Here's how the part is built. I have some questions about the finished solid (model axes, mm). Face numbers are marked on the shaded views. A direction names the side the tool comes from. Round coordinates to 2 decimals unless told otherwise and drop trailing zeros. Order: outer loops, then holes, each group sorted by start corner. A loop starts at its lowest first (then second) coordinate and runs counter-clockwise, first axis right, second up. Notation, with made-up numbers: M 48,63.25 L 59,63.25 A9 cw 59,74.25 Z; hole C -27,-20 d3. An arc over 180 degrees is marked long. Use one line per item in the form item = value. Start each with the question number.
```python
from build123d import *

# Parameters (mm, degrees)
SKETCH1_R                = 34.925
BOSS_EXTRUDE2_DEPTH      = 12.7
CUT_EXTRUDE3_START       = -25.4
CUT_EXTRUDE3_DEPTH       = 25.4
FILLET1_R                = 1.27
FILLET2_R                = 1.27
CIRPATTERN2_COUNT        = 20
FILLET1_OF_CIRPATTERN2_R = 1.27
FILLET2_OF_CIRPATTERN2_R = 1.27
CUT_EXTRUDE4_DEPTH       = 51.660303503
CUT_EXTRUDE4_DEPTH_BACK  = 51.660303503
SKETCH1_4_R              = 2.54
BOSS_EXTRUDE3_DEPTH      = 5.08


# Read off the part's stored shape, not the designer's step: Cut-Extrude3
with BuildPart() as part:
    # Sketch1 → Boss-Extrude2 (new, symmetric)
    with BuildSketch(Plane.XY):
        Circle(SKETCH1_R)
    extrude(amount=BOSS_EXTRUDE2_DEPTH, both=True)

    # Cut-Extrude3 outline → Cut-Extrude3 (cut)
    with BuildSketch(Plane.XY.offset(12.7).offset(CUT_EXTRUDE3_START)):
        with BuildLine():
            ThreePointArc((-4.143363091, 34.678353007), (-2.305797051, 31.157002463), (-1.526035224, 27.262322746))
            ThreePointArc((-1.526035224, 27.262322746), (0, 27.305), (1.526035224, 27.262322746))
            ThreePointArc((1.526035224, 27.262322746), (2.305797051, 31.157002463), (4.143363091, 34.678353007))
            ThreePointArc((4.143363091, 34.678353007), (0, 34.925), (-4.143363091, 34.678353007))
        make_face()
    cut_extrude3 = extrude(amount=CUT_EXTRUDE3_DEPTH, mode=Mode.SUBTRACT)

    # Fillet1
    fillet1_edges = [part.edges().sort_by_distance(p)[0] for p in [
        (-1.526035224, 27.262322746, 0),
    ]]
    fillet(fillet1_edges, radius=FILLET1_R)

    # Fillet2
    fillet2_edges = [part.edges().sort_by_distance(p)[0] for p in [
        (1.526035224, 27.262322746, 0),
    ]]
    fillet(fillet2_edges, radius=FILLET2_R)

    # CirPattern2: Cut-Extrude3 ×20 about axis
    cirpattern2_axis = Axis((0, 0, 0), (0, 0, 1))
    for i in range(1, CIRPATTERN2_COUNT):
        add(cut_extrude3.rotate(cirpattern2_axis, i * 360 / CIRPATTERN2_COUNT), mode=Mode.SUBTRACT)

    # Fillet1 of CirPattern2
    fillet1_of_cirpattern2_edges = [part.edges().sort_by_distance(p)[0] for p in [
        (-9.875866779, 25.456438879, 0),
        (-17.258979684, 21.158701409, 0),
        (-22.952663407, 14.789802823, 0),
        (-26.399580515, 6.973175291, 0),
        (-27.262322746, -1.526035224, 0),
        (-25.456438879, -9.875866779, 0),
        (-21.158701409, -17.258979684, 0),
        (-14.789802823, -22.952663407, 0),
        (-6.973175291, -26.399580515, 0),
        (1.526035224, -27.262322746, 0),
        (9.875866779, -25.456438879, 0),
        (17.258979684, -21.158701409, 0),
        (22.952663407, -14.789802823, 0),
        (26.399580515, -6.973175291, 0),
        (27.262322746, 1.526035224, 0),
        (25.456438879, 9.875866779, 0),
        (21.158701409, 17.258979684, 0),
        (14.789802823, 22.952663407, 0),
        (6.973175291, 26.399580515, 0),
    ]]
    fillet(fillet1_of_cirpattern2_edges, radius=FILLET1_OF_CIRPATTERN2_R)

    # Fillet2 of CirPattern2
    fillet2_of_cirpattern2_edges = [part.edges().sort_by_distance(p)[0] for p in [
        (-6.973175291, 26.399580515, 0),
        (-14.789802823, 22.952663407, 0),
        (-21.158701409, 17.258979684, 0),
        (-25.456438879, 9.875866779, 0),
        (-27.262322746, 1.526035224, 0),
        (-26.399580515, -6.973175291, 0),
        (-22.952663407, -14.789802823, 0),
        (-17.258979684, -21.158701409, 0),
        (-9.875866779, -25.456438879, 0),
        (-1.526035224, -27.262322746, 0),
        (6.973175291, -26.399580515, 0),
        (14.789802823, -22.952663407, 0),
        (21.158701409, -17.258979684, 0),
        (25.456438879, -9.875866779, 0),
        (27.262322746, -1.526035224, 0),
        (26.399580515, 6.973175291, 0),
        (22.952663407, 14.789802823, 0),
        (17.258979684, 21.158701409, 0),
        (9.875866779, 25.456438879, 0),
    ]]
    fillet(fillet2_of_cirpattern2_edges, radius=FILLET2_OF_CIRPATTERN2_R)

    # Sketch1<4> → Cut-Extrude4 (cut, two sides: drawn at the far end of the back side and taken through both)
    with BuildSketch(Plane.XY.offset(-CUT_EXTRUDE4_DEPTH_BACK)):
        Circle(SKETCH1_4_R)
    extrude(amount=CUT_EXTRUDE4_DEPTH + CUT_EXTRUDE4_DEPTH_BACK, mode=Mode.SUBTRACT)

    # Sketch3 → Boss-Extrude3 (add)
    with BuildSketch(Plane.XY.offset(12.7)):
        Polygon((12.634064431, 0), (6.317032216, 10.941420751), (-6.317032216, 10.941420751), (-12.634064431, 0), (-6.317032216, -10.941420751), (6.317032216, -10.941420751), align=None)
    extrude(amount=BOSS_EXTRUDE3_DEPTH)


solid = part.part
```
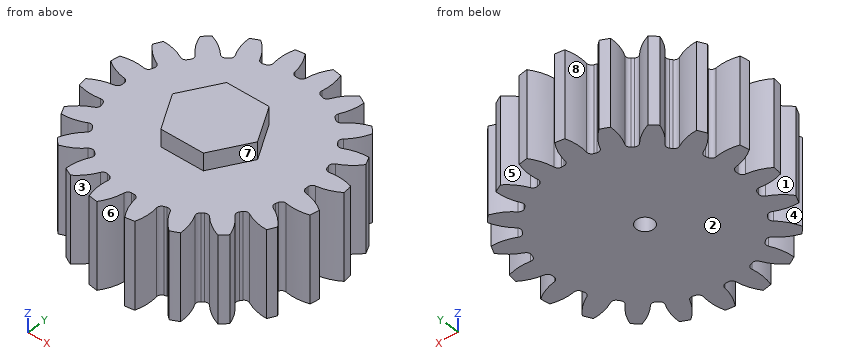
1) If we section it at B-B on y = 20: Write out the boundary of the cut face in (x, z).
2) If I drill on line 1 (Y direction, x = 0, z = 0) (3 decimals); line 2 (Y direction, x = -31, z = -8), over which ranges is the centre line in solid material (lowest first)?
3) If we section it at A-A on z = 14.5: Write out the boundary of the cut face in (x, y).
4) If we mould it in two halves opening along X, with no side actions, what happens to the marked faces 1, 2 and 3? For each: +X half, -X half, draft (parallel to the pull), parting line (faces both ways), or undercut.
5) Will these pins go through, and if not, where does the flat tip stop? pin 1 Ø4 at (x, z) = (3, 5.5) entering from -Y; pin 2 Ø1.5 at (x, z) = (1.5, 14.5) entering from +Y; pin 3 Ø4 at (x, y) = (0, 0.5) entering from -Z; pin 4 Ø1 at (y, z) = (6, 8) entering from -X.
6) On a 3-axis mill with a long thin cutter (end or side, diameter ignored), from which of +Z, -Z, +X, -X, +Y, -Y can I reach the whole of each face in a straight line? I mean the marked faces 4, 5, 6, 7 and 8. Say none if no direction works.
Completed:
q1.outline = M -23.73,-12.7 L 23.73,-12.7 L 23.73,12.7 L -23.73,12.7 Z
q2.line_1 = -27.305 to -2.54, 2.54 to 27.305
q2.line_2 = -16.09 to -13.78, -7.4 to -2.25, 2.25 to 7.4, 13.78 to 16.09
q3.outline = M -12.63,0 L -6.32,-10.94 L 6.32,-10.94 L 12.63,0 L 6.32,10.94 L -6.32,10.94 Z
q4.face_1 = -X half
q4.face_2 = draft
q4.face_3 = undercut
q5.pin_1 = -34.68
q5.pin_2 = 10.94
q5.pin_3 = 12.7
q5.pin_4 = -34.49
q6.face_4 = +Z, -Z, -X
q6.face_5 = +Z, -Z, +Y
q6.face_6 = +Z, -Z, -Y
q6.face_7 = +Z, +X, -Y
q6.face_8 = +Z, -Z
